```python
from build123d import *

# Parameters (mm, degrees)
BASE_FLANGE3_DEPTH             = 406.4
SKETCH10_R                     = 1.4478
CUT_EXTRUDE3_DEPTH             = 594.198769469
SKETCH11_R                     = 2.032
CUT_EXTRUDE4_DEPTH             = 594.139546967
F_7_16_0_4375_DIAMETER_HOLE1_D = 11.1125


# Sheet-metal steps are written as plain solids
with BuildPart() as part:
    # Sketch1 → Base-Flange3 (new body)
    with BuildSketch(Plane.XY):
        with BuildLine():
            Line((431.8, 16.51), (431.8, 2.4384))
            ThreePointArc((431.8, 2.4384), (431.085809175, 0.714190825), (429.3616, 0))
            Line((429.3616, 0), (2.4384, 0))
            ThreePointArc((2.4384, 0), (0.714190825, 0.714190825), (0, 2.4384))
            Line((0, 2.4384), (0, 16.51))
            Line((0, 16.51), (2.286, 16.51))
            Line((2.286, 16.51), (2.286, 2.4384))
            ThreePointArc((2.286, 2.4384), (2.330636927, 2.330636927), (2.4384, 2.286))
            Line((2.4384, 2.286), (429.3616, 2.286))
            ThreePointArc((429.3616, 2.286), (429.469363073, 2.330636927), (429.514, 2.4384))
            Line((429.514, 2.4384), (429.514, 16.51))
            Line((429.514, 16.51), (431.8, 16.51))
        make_face()
    extrude(amount=BASE_FLANGE3_DEPTH)

    # Sketch10 → Cut-Extrude3 (cut, through all)
    with BuildSketch(Plane(origin=(431.8, 0, 0), x_dir=(0, 0, -1), z_dir=(1, 0, 0))):
        with Locations((-31.75, 10.16)):
            Circle(SKETCH10_R)
        with Locations((-146.05, 10.16)):
            Circle(SKETCH10_R)
        with Locations((-260.35, 10.16)):
            Circle(SKETCH10_R)
        with Locations((-374.65, 10.16)):
            Circle(SKETCH10_R)
    extrude(amount=-CUT_EXTRUDE3_DEPTH, mode=Mode.SUBTRACT)

    # Sketch11 → Cut-Extrude4 (cut, through all)
    with BuildSketch(Plane(origin=(0, 2.286, 0), x_dir=(-1, 0, 0), z_dir=(0, 1, 0))):
        with Locations(Location((-406.4, 397.002, 0), (0, 0, 90))):
            Circle(SKETCH11_R)
        with Locations(Location((-279.4, 397.002, 0), (0, 0, 90))):
            Circle(SKETCH11_R)
        with Locations(Location((-152.4, 397.002, 0), (0, 0, 90))):
            Circle(SKETCH11_R)
        with Locations(Location((-25.4, 397.002, 0), (0, 0, 90))):
            Circle(SKETCH11_R)
        with Locations(Location((-406.4, 9.398, 0), (0, 0, 90))):
            Circle(SKETCH11_R)
        with Locations(Location((-279.4, 9.398, 0), (0, 0, 90))):
            Circle(SKETCH11_R)
        with Locations(Location((-152.4, 9.398, 0), (0, 0, 90))):
            Circle(SKETCH11_R)
        with Locations(Location((-25.4, 9.398, 0), (0, 0, 90))):
            Circle(SKETCH11_R)
    extrude(amount=-CUT_EXTRUDE4_DEPTH, mode=Mode.SUBTRACT)

    # 7/16 (0.4375) Diameter Hole1 (through all)
    with Locations(Plane(origin=(0, 2.286, 0), x_dir=(1, 0, 0), z_dir=(0, 1, 0))):
        with Locations((25.4, -31.75), (406.4, -31.75), (406.4, -374.65), (25.4, -374.65)):
            Hole(F_7_16_0_4375_DIAMETER_HOLE1_D / 2)


solid = part.part
```
Geometry check sheet. Reference: the model listing, model coordinates, mm. A direction names the side the tool comes from. Coordinates: 2 decimals unless noted, no trailing zeros. Order: outer loops, then holes, each group sorted by start corner. A loop starts at its lowest first (then second) coordinate and runs counter-clockwise, first axis right, second up.
Q1. Sectioned sample at B-B on z = 105. Record the cut outline in (x, y), and give its area (3 significant figures).
Reply:
outline: (0, 2.44) arc R2.44 ccw to (2.44, 0) - (429.36, 0) arc R2.44 ccw to (431.8, 2.44) - (431.8, 16.51) - (429.51, 16.51) - (429.51, 2.44) arc R0.15 cw to (429.36, 2.29) - (2.44, 2.29) arc R0.15 cw to (2.29, 2.44) - (2.29, 16.51) - (0, 16.51) - close
area: 1,050 mm2
Q2. Draft check along Z on faces 1 (the face through (217, 2, 0)), 2 (the face through (407.604, 1.127, 380.074)), 3 (the face through (0, 9, 200)). Enter one of: released by +Z, released by -Z, zero draft, split by the parting line, or undercut.
Reply:
face 1: released by -Z
face 2: undercut
face 3: zero draft
Q3. Depth check by flat-ended pin: pin 1 Ø3.5 at (y, z) = (10.16, 31.75) entering from -X; pin 2 Ø5.5 at (x, z) = (152.4, 397.002) entering from +Y. Enter the tip coordinate at first touch or a pass-through.
Reply:
pin 1: stops at x = 0
pin 2: stops at y = 2.29
Q4. Sectioned sample at A-A on y = 5.75. Record the cut outline in (x, z), and give its area (3 significant figures).
Reply:
outline: (0, 0) - (2.29, 0) - (2.29, 406.4) - (0, 406.4) - close; (429.51, 0) - (431.8, 0) - (431.8, 406.4) - (429.51, 406.4) - close
area: 1,860 mm2
Q5. Tool access check on faces 4 (the face through (431.8, 10, 200)), 5 (the face through (429.514, 9, 200)). Record the directions out of +Z, -Z, +X, -X, +Y, -Y that give a thin tool (end or side, any length) a straight path to the whole face; none if there is none.
Reply:
face 4: +Z, -Z, +X, +Y, -Y
face 5: +Z, -Z, +Y
Q6. Thickness scan on probe 1 along Z at (x, y) = (279.4, 1.05); probe 2 along X at (y, z) = (4, 56); probe 3 along Y at (x, z) = (290.5, 353). Record the ranges inside material, lowest first.
Reply:
probe 1: z = 0 to 7.37, 11.43 to 394.97, 399.03 to 406.4
probe 2: x = 0 to 2.29, 429.51 to 431.8
probe 3: y = 0 to 2.29
Q7. Sectioned sample at C-C on x = 391. Record the cut outline in (y, z).
Reply:
outline: (0, 0) - (2.29, 0) - (2.29, 406.4) - (0, 406.4) - close
